Read the model definition and answer for the solid it produces. Units are mm, in the model's axes. A direction names the side the tool comes from. Coordinates: 2 decimals unless noted, no trailing zeros. Order: outer loops, then holes, each group sorted by start corner. A loop starts at its lowest first (then second) coordinate and runs counter-clockwise, first axis right, second up. Notation, with made-up numbers: M 72.25,12 L 76.25,12 A20 ccw 76.25,33 Z; hole C -9,-28.75 d1. An arc over 180 degrees is marked long. Write each question's results on one line, items separated by ' | '.
```python
from build123d import *
from build123d.topology import SkipClean

# Parameters (mm, degrees)
SKETCH_1_R          = 30
SKETCH_1_R_2        = 3
EXTRUDE_1_DEPTH     = 30
EXTRUDE_START       = -20
SKETCH_2_R          = 40
EXTRUDE_2_DEPTH     = 20
CUT_EXTRUDE_START   = -20
CUT_EXTRUDE_1_DEPTH = 20
EXTRUDE_START_2     = -30
SKETCH_4_R          = 3
SKETCH_4_R_2        = 2
EXTRUDE_4_DEPTH     = 30


with BuildPart() as part:
    # 草图1 → 凸台-拉伸1 (new body)
    with BuildSketch(Plane(origin=(0, 0, 0), x_dir=(1, 0, 0), z_dir=(0, 1, 0))):
        with Locations(Location((0, 0, 0), (0, 0, 270))):
            Circle(SKETCH_1_R)
        with Locations(Location((-17.25, 0, 0), (0, 0, 270))):
            Circle(SKETCH_1_R_2, mode=Mode.SUBTRACT)
        with Locations(Location((-8.625, 14.938938215, 0), (0, 0, 270))):
            Circle(SKETCH_1_R_2, mode=Mode.SUBTRACT)
        with Locations(Location((8.625, 14.938938215, 0), (0, 0, 270))):
            Circle(SKETCH_1_R_2, mode=Mode.SUBTRACT)
        with Locations(Location((17.25, 0, 0), (0, 0, 270))):
            Circle(SKETCH_1_R_2, mode=Mode.SUBTRACT)
        with Locations(Location((8.625, -14.938938215, 0), (0, 0, 270))):
            Circle(SKETCH_1_R_2, mode=Mode.SUBTRACT)
        with Locations(Location((-8.625, -14.938938215, 0), (0, 0, 270))):
            Circle(SKETCH_1_R_2, mode=Mode.SUBTRACT)
    extrude(amount=EXTRUDE_1_DEPTH)

    # 草图2 → 凸台-拉伸2 (add)
    with BuildSketch(Plane(origin=(0, 30, 0), x_dir=(1, 0, 0), z_dir=(0, 1, 0)).offset(EXTRUDE_START)):
        with Locations(Location((0, 0, 0), (0, 0, 270))):
            Circle(SKETCH_2_R)
        with BuildLine():
            ThreePointArc((2.996247653, 29.85), (21.213203436, 21.213203436), (29.85, 2.996247653))
            ThreePointArc((29.85, 2.996247653), (32.067607313, 2.173706512), (33, 0))
            ThreePointArc((33, 0), (32.067607313, -2.173706512), (29.85, -2.996247653))
            ThreePointArc((29.85, -2.996247653), (21.213203436, -21.213203436), (2.996247653, -29.85))
            ThreePointArc((2.996247653, -29.85), (2.999061767, -29.924976537), (3, -30))
            ThreePointArc((3, -30), (-0.075023463, -32.999061767), (-2.996247653, -29.85))
            ThreePointArc((-2.996247653, -29.85), (-21.213203436, -21.213203436), (-29.85, -2.996247653))
            ThreePointArc((-29.85, -2.996247653), (-33, 0), (-29.85, 2.996247653))
            ThreePointArc((-29.85, 2.996247653), (-21.213203436, 21.213203436), (-2.996247653, 29.85))
            ThreePointArc((-2.996247653, 29.85), (-0.075023463, 32.999061767), (3, 30))
            ThreePointArc((3, 30), (2.999061767, 29.924976537), (2.996247653, 29.85))
        make_face(mode=Mode.SUBTRACT)
    extrude(amount=EXTRUDE_2_DEPTH)

    # 草图3 → 切除-拉伸1 (cut)
    with SkipClean():  # the faces are left unmerged after this step: merging them gives an invalid solid
        with BuildSketch(Plane(origin=(0, 30, 0), x_dir=(1, 0, 0), z_dir=(0, 1, 0)).offset(CUT_EXTRUDE_START)):
            with BuildLine():
                ThreePointArc((29.85, -2.996247653), (29.962476533, -1.5), (30, 0))
                ThreePointArc((30, 0), (29.962476533, 1.5), (29.85, 2.996247653))
                ThreePointArc((29.85, 2.996247653), (27, 0), (29.85, -2.996247653))
            make_face()
            with BuildLine():
                ThreePointArc((29.85, 2.996247653), (29.962476533, 1.5), (30, 0))
                ThreePointArc((30, 0), (29.962476533, -1.5), (29.85, -2.996247653))
                ThreePointArc((29.85, -2.996247653), (32.067607313, -2.173706512), (33, 0))
                ThreePointArc((33, 0), (32.067607313, 2.173706512), (29.85, 2.996247653))
            make_face()
            with BuildLine():
                ThreePointArc((-2.996247653, 29.85), (0, 27), (2.996247653, 29.85))
                ThreePointArc((2.996247653, 29.85), (0, 30), (-2.996247653, 29.85))
            make_face()
            with BuildLine():
                ThreePointArc((-2.996247653, 29.85), (0, 30), (2.996247653, 29.85))
                ThreePointArc((2.996247653, 29.85), (2.999061767, 29.924976537), (3, 30))
                ThreePointArc((3, 30), (-0.075023463, 32.999061767), (-2.996247653, 29.85))
            make_face()
            with BuildLine():
                ThreePointArc((3, -30), (2.999061767, -29.924976537), (2.996247653, -29.85))
                ThreePointArc((2.996247653, -29.85), (0, -30), (-2.996247653, -29.85))
                ThreePointArc((-2.996247653, -29.85), (-0.075023463, -32.999061767), (3, -30))
            make_face()
            with BuildLine():
                ThreePointArc((-2.996247653, -29.85), (0, -30), (2.996247653, -29.85))
                ThreePointArc((2.996247653, -29.85), (0, -27), (-2.996247653, -29.85))
            make_face()
            with BuildLine():
                ThreePointArc((-27, 0), (-27.826293488, 2.067607313), (-29.85, 2.996247653))
                ThreePointArc((-29.85, 2.996247653), (-30, 0), (-29.85, -2.996247653))
                ThreePointArc((-29.85, -2.996247653), (-27.826293488, -2.067607313), (-27, 0))
            make_face()
            with BuildLine():
                ThreePointArc((-29.85, -2.996247653), (-30, 0), (-29.85, 2.996247653))
                ThreePointArc((-29.85, 2.996247653), (-33, 0), (-29.85, -2.996247653))
            make_face()
        extrude(amount=CUT_EXTRUDE_1_DEPTH, mode=Mode.SUBTRACT)

    # 草图4 → 凸台-拉伸4 (add)
    # profile 1 of 6: a face of its own
    with SkipClean():  # the faces are left unmerged after this step: merging them gives an invalid solid
        with BuildSketch(Plane(origin=(0, 30, 0), x_dir=(1, 0, 0), z_dir=(0, 1, 0)).offset(EXTRUDE_START_2)):
            with Locations((17.25, 0)):
                Circle(SKETCH_4_R)
            with Locations(Location((17.25, 0, 0), (0, 0, 270))):
                Circle(SKETCH_4_R_2, mode=Mode.SUBTRACT)
        # profile 2 of 6: a face of its own
        with BuildSketch(Plane(origin=(0, 30, 0), x_dir=(1, 0, 0), z_dir=(0, 1, 0)).offset(EXTRUDE_START_2)):
            with Locations((8.625, 14.938938215)):
                Circle(SKETCH_4_R)
            with Locations(Location((8.625, 14.938938215, 0), (0, 0, 270))):
                Circle(SKETCH_4_R_2, mode=Mode.SUBTRACT)
        # profile 3 of 6: a face of its own
        with BuildSketch(Plane(origin=(0, 30, 0), x_dir=(1, 0, 0), z_dir=(0, 1, 0)).offset(EXTRUDE_START_2)):
            with Locations((8.625, -14.938938215)):
                Circle(SKETCH_4_R)
            with Locations(Location((8.625, -14.938938215, 0), (0, 0, 270))):
                Circle(SKETCH_4_R_2, mode=Mode.SUBTRACT)
        # profile 4 of 6: a face of its own
        with BuildSketch(Plane(origin=(0, 30, 0), x_dir=(1, 0, 0), z_dir=(0, 1, 0)).offset(EXTRUDE_START_2)):
            with Locations((-8.625, 14.938938215)):
                Circle(SKETCH_4_R)
            with Locations(Location((-8.625, 14.938938215, 0), (0, 0, 270))):
                Circle(SKETCH_4_R_2, mode=Mode.SUBTRACT)
        # profile 5 of 6: a face of its own
        with BuildSketch(Plane(origin=(0, 30, 0), x_dir=(1, 0, 0), z_dir=(0, 1, 0)).offset(EXTRUDE_START_2)):
            with Locations((-8.625, -14.938938215)):
                Circle(SKETCH_4_R)
            with Locations(Location((-8.625, -14.938938215, 0), (0, 0, 270))):
                Circle(SKETCH_4_R_2, mode=Mode.SUBTRACT)
        # profile 6 of 6: a face of its own
        with BuildSketch(Plane(origin=(0, 30, 0), x_dir=(1, 0, 0), z_dir=(0, 1, 0)).offset(EXTRUDE_START_2)):
            with Locations((-17.25, 0)):
                Circle(SKETCH_4_R)
            with Locations(Location((-17.25, 0, 0), (0, 0, 270))):
                Circle(SKETCH_4_R_2, mode=Mode.SUBTRACT)
        extrude(amount=EXTRUDE_4_DEPTH)


solid = part.part
```
(1) Given pin 1 (3.5 mm diameter, centred on x = -29, z = 0.5, fed in from +Y); pin 2 (2.5 mm diameter, centred on x = -17.25, z = 0, fed in from -Y); pin 3 (10 mm diameter, centred on y = 16.5, z = 0, fed in from +X); pin 4 (6 mm diameter, centred on x = -27.5, y = 12.5, fed in from -Z), each flat-ended and moving along its own axis, determine where each tip first touches the part or whether it passes through.
Conclusion:
pin 1: y = 10 | pin 2: through | pin 3: x = 40 | pin 4: z = -31.62
(2) The part is cut by section B-B, the plane y = 18.75. Count the separate pieces of the cut face and the enclosed holes in it, then the cut area to 3 significant figures.
Conclusion:
separate pieces: 1 | enclosed holes: 10 | area: 4,840 mm²
(3) The part is cut by section C-C, the plane z = 11. Write down the section's boundary in (x, y).
Conclusion:
outline: M -38.46,10 L -27.91,10 L -27.91,0 L 27.91,0 L 27.91,10 L 38.46,10 L 38.46,30 L -38.46,30 Z
(4) The part is cut by section D-D, the plane x = -24. Write down the section's boundary in (y, z).
Conclusion:
outline: M 0,-18 L 10,-18 L 10,-32 L 30,-32 L 30,32 L 10,32 L 10,18 L 0,18 Z
(5) Straight lines are drawn through the part: line 1 (X direction, y = 8.5, z = 0); line 2 (Z direction, x = 8.5, y = 3.75); line 3 (Z direction, x = 8, y = 19.75). For each, find the intervals that lie inside material, in ascending order.
Conclusion:
line 1: -30 to -19.25, -15.25 to 15.25, 19.25 to 30 | line 2: -28.77 to -16.94, -12.94 to 12.94, 16.94 to 28.77 | line 3: -39.19 to -16.84, -13.04 to 13.04, 16.84 to 39.19
(6) For faces 4 (the flat face through (0, 10, -29)), 5 (the flat face through (0, 0, 0)), determine the directions among +Z, -Z, +X, -X, +Y, -Y from which every point of the face is accessible in a straight line to the end or side of a thin tool.
Conclusion:
face 4: +Y | face 5: +Z, -Z, +X, -X, -Y
(7) The part is cut by section A-A, the plane x = 17.25. Write down the section's boundary in (y, z), then the cut area to 3 significant figures.
Conclusion:
outline: M 0,-24.54 L 10,-24.54 L 10,-36.09 L 30,-36.09 L 30,-2 L 0,-2 Z; M 0,2 L 30,2 L 30,36.09 L 10,36.09 L 10,24.54 L 0,24.54 Z | area: 1,810 mm²
(8) The mould has two halves that part along Z. Classify faces 1 (the flat face through (-29, 10, 9)), 2 (the cylindrical face through (-11.49, 4.93, 27.712)), 3 (the flat face through (0, 10, 29)): pulls with the +Z half, pulls with the -Z half, needs draft (parallel to the pull), parting line crosses it, or undercut.
Conclusion:
face 1: needs draft | face 2: parting line crosses it | face 3: undercut
